from build123d import *

# Parameters (mm, degrees)
F0_R     = 17.5
F1_DEPTH = 129
F2_SIZE  = 2
F3_R     = 22
F4_DEPTH = 6
F5_SIZE  = 2
F6_W     = 7
F6_H     = 17.894253
F7_DEPTH = 25


with BuildPart() as f1:
    # F0 (on Right) → F1 (new body)
    with BuildSketch(Plane.YZ):
        Circle(F0_R)
    extrude(amount=F1_DEPTH)

    # F2
    f2_edges = [f1.edges().sort_by_distance(p)[0] for p in [
        (129, -17.5, 0),
    ]]
    chamfer(f2_edges, length=F2_SIZE)

    # F3 (on face) → F4 (join)
    with BuildSketch(Plane(origin=(0, 0, 0), x_dir=(0, -1, 0), z_dir=(-1, 0, 0))):
        Circle(F3_R)
    extrude(amount=F4_DEPTH)

    # F5
    f5_edges = [f1.edges().sort_by_distance(p)[0] for p in [
        (-6, 22, 0),
    ]]
    chamfer(f5_edges, length=F5_SIZE)

    # F6 (on Front) → F7 (cut, symmetric)
    with BuildSketch(Plane.XZ):
        with Locations((115.5, -17.947126)):
            Rectangle(F6_W, F6_H)
    extrude(amount=F7_DEPTH, both=True, mode=Mode.SUBTRACT)


solid = f1.part
Model file for the job. Use its own axes, mm. A direction names the side the tool comes from. Round coordinates to 2 decimals unless told otherwise and drop trailing zeros. Order: outer loops, then holes, each group sorted by start corner. A loop starts at its lowest first (then second) coordinate and runs counter-clockwise, first axis right, second up.
(1) Pull direction X, two halves, no side cores. Call faces 1 (the face through (62.611, -13.887, -10.648)), 2 (the face through (112, 0, -12)), 3 (the face through (119, 0, -12)), 4 (the face through (129, 0, 0)): released by +X, released by -X, zero draft, split by the parting line, or undercut.
(2) Drill centre lines: line 1 (X direction, y = -1.5, z = -16.5); line 2 (X direction, y = -3.5, z = 17.5); line 3 (X direction, y = -10, z = -13). Where is each one in solid material? Low to high.
(3) 3-axis set-ups, long thin cutter, end or side, ignore diameter. For faces 5 (the face through (115, 0, -9)), 6 (the face through (0, 15, -10)), 7 (the face through (-6, 0, 0)): which of +Z, -Z, +X, -X, +Y, -Y reach the whole face in a straight line?
(4) Band-saw the part on A-A (z = 0). List the corners of the cut face in (x, y).
(5) Band-saw the part on B-B (y = 0). List the corners of the cut face in (x, z), then the cut area to 3 significant figures.
(6) Pin check, flat tips, straight feed: pin 1 (12 mm diameter, centred on x = 39, z = 15, fed in from +Y); pin 2 (1 mm diameter, centred on x = 91, y = -9, fed in from -Z); pin 3 (6 mm diameter, centred on x = 113.5, y = -3, fed in from -Z). Stop position of each tip, or through.
Verdict:
1. face 1: zero draft
1. face 2: undercut
1. face 3: undercut
1. face 4: released by +X
2. line 1: x = -6 to 112, 119 to 127.93
2. line 2: x = -6 to 0
2. line 3: x = -6 to 112, 119 to 128.1
3. face 5: -Z, +Y, -Y
3. face 6: +X
3. face 7: +Z, -Z, -X, +Y, -Y
4. outline: (-6, -20) - (-4, -22) - (0, -22) - (0, -17.5) - (127, -17.5) - (129, -15.5) - (129, 15.5) - (127, 17.5) - (0, 17.5) - (0, 22) - (-4, 22) - (-6, 20) - close
5. outline: (-6, -20) - (-4, -22) - (0, -22) - (0, -17.5) - (112, -17.5) - (112, -9) - (119, -9) - (119, -17.5) - (127, -17.5) - (129, -15.5) - (129, 15.5) - (127, 17.5) - (0, 17.5) - (0, 22) - (-4, 22) - (-6, 20) - close
5. area: 4,710 mm2
6. pin 1: stops at y = 15.01
6. pin 2: stops at z = -15.3
6. pin 3: stops at z = -17.5
